```python
from build123d import *

# Parameters (mm, degrees)
F0_W     = 20.6
F0_H     = 4
F1_DEPTH = 13.4
F2_W     = 4.6
F2_H     = 4
F3_DEPTH = 4.2
F4_R     = 1.3
F5_DEPTH = 25
F6_R     = 1.99999


# Not quite as in the source:
# - a fillet or chamfer is up to 0.001 mm smaller than in the source, because OpenCascade refuses the exact size


with BuildPart() as f1:
    # F0 (on Front) → F1 (new body)
    with BuildSketch(Plane.XZ):
        with Locations((-17.0743378759, 29.5677930117)):
            Rectangle(F0_W, F0_H)
    extrude(amount=F1_DEPTH)

    # F2 (on face) → F3 (join)
    with BuildSketch(Plane.YZ.offset(-6.7743378759)):
        with Locations((-8.9, 29.5677930117)):
            Rectangle(F2_W, F2_H)
    extrude(amount=F3_DEPTH)

    # F4 (on face) → F5 (cut)
    with BuildSketch(Plane.XZ.offset(11.2)):
        with Locations((-4.3743378759, 29.5677930117)):
            Circle(F4_R)
    extrude(amount=-F5_DEPTH, mode=Mode.SUBTRACT)

    # F6 (radius 2 in the source; OpenCascade refuses exactly that, so slightly less here)
    f6_edges = [f1.edges().sort_by_distance(p)[0] for p in [
        (-2.574338, -8.9, 31.567793),
        (-2.574338, -8.9, 27.567793),
    ]]
    fillet(f6_edges, radius=F6_R)

    # F7: F1 across face


with BuildPart() as f1_1:
    add(f1.part)
    add(f1.part.mirror(Plane(origin=(-17.0743378759, 0, 29.5677930117), x_dir=(1, 0, 0), z_dir=(0, 1, 0))))


solid = f1_1.part
```
Design review of the part built by this model. Coordinates are the model's own, in mm. A direction names the side the tool comes from. Give positions to 0.01 mm unless a question says otherwise; leave off trailing zeros. Order: outer loops, then holes, each group sorted by start corner. A loop starts at its lowest first (then second) coordinate and runs counter-clockwise, first axis right, second up. Notation, with made-up numbers: (31, 20) -> (50, 20) arc R23 cw to (50, 40) -> close; hole circle Ø2 at (-34, 28). An arc over 180 degrees is marked (long way). Write item = value, one per line. Start each with the question number.
(1) Mouldability with a two-part tool opening along X and no side actions: class faces 4 (the face through (-4.66, -8.93, 28.3)), 5 (the face through (-27.374, 0, 30)), 6 (the face through (-3.176, -8.868, 28.138)), 7 (the face through (-6, 11.2, 29)) as +X half, -X half, draft (parallel to the pull), parting line (faces both ways), or undercut.
(2) We need section D-D on y = 1.75. Write out the cut boundary in (x, z), plus the area to 3 significant figures.
(3) To check wall thickness, follow line 1 along X through (y, z) = (7.25, 29.6); line 2 along X through (y, z) = (-0.5, 29.75); line 3 along X through (y, z) = (8.25, 29.95). State the ranges of each line that lie inside material, in increasing order.
(4) For pin 1 (0.7 mm diameter, centred on y = -12, z = 30, fed in from +X); pin 2 (1.2 mm diameter, centred on x = -5, z = 30, fed in from -Y), all flat-tipped, find the tip position at first contact; note any pin that passes through.
(5) For faces 1 (the face through (-6, -6.6, 29)), 2 (the face through (-6.774, 12, 30)), 3 (the face through (-6.774, -12, 30)), list the 3-axis set-ups (+Z, -Z, +X, -X, +Y, -Y) from which the entire face can be reached by the end or side of a thin tool; tool diameter is ignored.
(6) We need section B-B on z = 28.7. Write out the cut boundary in (x, y).
(7) We need section C-C on z = 31.2. Write out the cut boundary in (x, y), plus the area to 3 significant figures.
(8) We need section A-A on x = -4.25. Write out the cut boundary in (y, z).
Numbers:
q1.face_4 = undercut
q1.face_5 = -X half
q1.face_6 = +X half
q1.face_7 = draft
q2.outline = (-27.37, 27.57) -> (-6.77, 27.57) -> (-6.77, 31.57) -> (-27.37, 31.57) -> close
q2.area = 82.4 mm^2
q3.line_1 = -27.37 to -5.67, -3.07 to -2.57
q3.line_2 = -27.37 to -6.77
q3.line_3 = -27.37 to -5.62, -3.13 to -2.61
q4.pin_1 = -6.77
q4.pin_2 = -11.2
q5.face_1 = +Z, -Z, +X
q5.face_2 = +Z, -Z, +X, +Y
q5.face_3 = +Z, -Z, +X, -Y
q6.outline = (-27.37, -13.4) -> (-6.77, -13.4) -> (-6.77, -11.2) -> (-5.34, -11.2) -> (-5.34, -6.6) -> (-6.77, -6.6) -> (-6.77, 6.6) -> (-5.34, 6.6) -> (-5.34, 11.2) -> (-6.77, 11.2) -> (-6.77, 13.4) -> (-27.37, 13.4) -> close; (-3.41, -11.2) -> (-2.77, -11.2) -> (-2.77, -6.6) -> (-3.41, -6.6) -> close; (-3.41, 6.6) -> (-2.77, 6.6) -> (-2.77, 11.2) -> (-3.41, 11.2) -> close
q7.outline = (-27.37, -13.4) -> (-6.77, -13.4) -> (-6.77, -11.2) -> (-3.42, -11.2) -> (-3.42, -6.6) -> (-6.77, -6.6) -> (-6.77, 6.6) -> (-3.42, 6.6) -> (-3.42, 11.2) -> (-6.77, 11.2) -> (-6.77, 13.4) -> (-27.37, 13.4) -> close
q7.area = 583 mm^2
q8.outline = (-11.2, 27.59) -> (-6.6, 27.59) -> (-6.6, 28.27) -> (-11.2, 28.27) -> close; (-11.2, 30.86) -> (-6.6, 30.86) -> (-6.6, 31.54) -> (-11.2, 31.54) -> close; (6.6, 27.59) -> (11.2, 27.59) -> (11.2, 28.27) -> (6.6, 28.27) -> close; (6.6, 30.86) -> (11.2, 30.86) -> (11.2, 31.54) -> (6.6, 31.54) -> close
